Here's how the part is built. I have some questions about the finished solid (model axes, mm). Coordinates: 2 decimals unless noted, no trailing zeros. Order: outer loops, then holes, each group sorted by start corner. A loop starts at its lowest first (then second) coordinate and runs counter-clockwise, first axis right, second up.
```python
from build123d import *

# Parameters (mm, degrees)
BOSS_EXTRUDE1_DEPTH  = 1.5
CUT_EXTRUDE1_DEPTH   = 114.470260421
FILLET1_R            = 1.5
M3_CLEARANCE_HOLE1_D = 3.2
M2_CLEARANCE_HOLE2_D = 2.2


with BuildPart() as part:
    # Sketch1 → Boss-Extrude1 (new body)
    with BuildSketch(Plane.XY):
        with BuildLine():
            Line((3, -23.5), (109, -23.5))
            ThreePointArc((109, -23.5), (110.414213562, -22.914213562), (111, -21.5))
            Line((111, -21.5), (111, 21.5))
            ThreePointArc((111, 21.5), (110.414213562, 22.914213562), (109, 23.5))
            Line((109, 23.5), (3, 23.5))
            ThreePointArc((3, 23.5), (0.878679656, 22.621320344), (0, 20.5))
            Line((0, 20.5), (0, -20.5))
            ThreePointArc((0, -20.5), (0.878679656, -22.621320344), (3, -23.5))
        make_face()
    extrude(amount=BOSS_EXTRUDE1_DEPTH)

    # Sketch2 → Cut-Extrude1 (cut, through all)
    with BuildSketch(Plane(origin=(0, 0, 0), x_dir=(-1, 0, 0), z_dir=(0, 0, -1))):
        with BuildLine():
            Line((-101, 19.5), (-101, 23.5))
            Line((-101, 23.5), (-109, 23.5))
            ThreePointArc((-109, 23.5), (-110.414213562, 22.914213562), (-111, 21.5))
            Line((-111, 21.5), (-111, 19.5))
            Line((-111, 19.5), (-101, 19.5))
        make_face()
        with BuildLine():
            Line((-101, -19.5), (-111, -19.5))
            Line((-111, -19.5), (-111, -21.5))
            ThreePointArc((-111, -21.5), (-110.414213562, -22.914213562), (-109, -23.5))
            Line((-109, -23.5), (-101, -23.5))
            Line((-101, -23.5), (-101, -19.5))
        make_face()
    extrude(amount=-CUT_EXTRUDE1_DEPTH, mode=Mode.SUBTRACT)

    # Fillet1
    fillet1_edges = [part.edges().sort_by_distance(p)[0] for p in [
        (101, 19.5, 0.75),
        (111, 19.5, 0.75),
        (101, 23.5, 0.75),
        (101, -23.5, 0.75),
        (111, -19.5, 0.75),
        (101, -19.5, 0.75),
    ]]
    fillet(fillet1_edges, radius=FILLET1_R)

    # M3 Clearance Hole1 (through all)
    with Locations(Plane.XY.offset(1.5)):
        with Locations((28.437, 3.0309), (28.437, -12.0821)):
            Hole(M3_CLEARANCE_HOLE1_D / 2)

    # M2 Clearance Hole2 (through all)
    with Locations(Plane.XY.offset(1.5)):
        with Locations((105.6, 9.525), (105.6, -8.525)):
            Hole(M2_CLEARANCE_HOLE2_D / 2)


solid = part.part
```
Q1. Will this pin go through, and if not, where does the flat tip stop? pin 1 (0.8 mm diameter, centred on y = 21.5, z = 0.5, fed in from +X).
Q2. We'd pull the mould along Y, two halves only. Please class faces 1 (the cylindrical face through (106.7, -8.5, 0.7)), 2 (the cylindrical face through (0.9, 22.64, 0.74)), 3 (the flat face through (55, 0, 1.5)): pulls with the +Y half, pulls with the -Y half, needs draft (parallel to the pull), parting line crosses it, or undercut.
Q3. If we section it at A-A on x = 105.6: Write out the boundary of the cut face in (y, z) (3 decimals).
Q4. I need wall thicknesses on L1, parallel to Y at x = 105.6, z = 0.7 (3 decimals); L2, parallel to X at y = 10, z = 0.4; L3, parallel to X at y = -13.5, z = 0.75. Which ranges of each line are inside material? Lowest first, please.
Q5. If we section it at B-B on z = 1.25: Write out the boundary of the cut face in (x, y) (3 decimals).
Reply:
1. pin 1: stops at x = 101
2. face 1: undercut
2. face 2: pulls with the +Y half
2. face 3: needs draft
3. outline: (-19.5, 0) - (-9.625, 0) - (-9.625, 1.5) - (-19.5, 1.5) - close; (-7.425, 0) - (8.425, 0) - (8.425, 1.5) - (-7.425, 1.5) - close; (10.625, 0) - (19.5, 0) - (19.5, 1.5) - (10.625, 1.5) - close
4. L1: y = -19.5 to -9.625, -7.425 to 8.425, 10.625 to 19.5
4. L2: x = 0 to 104.61, 106.59 to 111
4. L3: x = 0 to 27.7, 29.18 to 111
5. outline: (0, -20.5) arc R3 ccw to (3, -23.5) - (99.5, -23.5) arc R1.5 ccw to (101, -22) - (101, -21) arc R1.5 cw to (102.5, -19.5) - (109.5, -19.5) arc R1.5 ccw to (111, -18) - (111, 18) arc R1.5 ccw to (109.5, 19.5) - (102.5, 19.5) arc R1.5 cw to (101, 21) - (101, 22) arc R1.5 ccw to (99.5, 23.5) - (3, 23.5) arc R3 ccw to (0, 20.5) - close; hole circle Ø3.2 at (28.437, -12.082); hole circle Ø3.2 at (28.437, 3.031); hole circle Ø2.2 at (105.6, -8.525); hole circle Ø2.2 at (105.6, 9.525)
